from build123d import *
from OCP.BRepFilletAPI import BRepFilletAPI_MakeChamfer

# Parameters (mm, degrees)
EXTRUDE_1_DEPTH  = 8.6
CHAMFER_1_SIZE   = 0.5
CHAMFER_1_SIZE2  = 0.866025404
CHAMFER_2_SIZE   = 0.142054737
CHAMFER_2_SIZE_2 = 0.2


with BuildPart() as part:
    # 草图1 → 凸台-拉伸1 (new body)
    with BuildSketch(Plane.XY):
        with BuildLine():
            Line((-128.840361964, -116.659683115), (-127.425332489, -116.659683115))
            ThreePointArc((-127.425332489, -116.659683115), (-132.090361964, -126.69001389), (-136.755391439, -116.659683115))
            Line((-136.755391439, -116.659683115), (-135.340361964, -116.659683115))
            ThreePointArc((-135.340361964, -116.659683115), (-132.090361964, -125.69001389), (-128.840361964, -116.659683115))
        make_face()
    extrude(amount=EXTRUDE_1_DEPTH)

    # 倒角1: one chamfer whose edges measure the first distance from different faces: ONE call of the kernel's chamfer builder (chamfer() names one face for all edges)
    chamfer_1_edges_1 = [part.edges().sort_by_distance(p)[0] for p in [
        (-136.047876701, -116.659683115, 8.6),
    ]]
    chamfer_1_side_1 = [part.faces().sort_by_distance(p)[0] for p in [
        (-136.047876701, -116.659683115, 4.3),
    ]]
    chamfer_1_edges_2 = [part.edges().sort_by_distance(p)[0] for p in [
        (-128.132847227, -116.659683115, 8.6),
    ]]
    chamfer_1_side_2 = [part.faces().sort_by_distance(p)[0] for p in [
        (-128.132847227, -116.659683115, 4.3),
    ]]
    chamfer_1 = BRepFilletAPI_MakeChamfer(part.part.solid().wrapped)
    for e in chamfer_1_edges_1:
        chamfer_1.Add(CHAMFER_1_SIZE, CHAMFER_1_SIZE2, e.wrapped, chamfer_1_side_1[0].wrapped)  # the first distance lies on this face
    for e in chamfer_1_edges_2:
        chamfer_1.Add(CHAMFER_1_SIZE, CHAMFER_1_SIZE2, e.wrapped, chamfer_1_side_2[0].wrapped)  # the first distance lies on this face
    add(Compound.cast(chamfer_1.Shape()), mode=Mode.REPLACE)

    # 倒角2
    # the kernel refuses this chamfer: 0.2, 0.142054737 mm, written as the material it takes off along each edge
    with BuildSketch(Plane(origin=(-135.340361964, -116.659683115, -0.524920029), x_dir=(-0.7577457918240572, -0.6525498563120925, 0), z_dir=(0, 0, 1))) as chamfer_2_piece_1:
        with BuildLine():
            Line((0.204125918, 0), (CHAMFER_2_SIZE * 0.757745791973, -CHAMFER_2_SIZE * 0.65254985644))
            Line((CHAMFER_2_SIZE * 0.757745791973, -CHAMFER_2_SIZE * 0.65254985644), (0, 0))
            ThreePointArc((0, 0), (0.104949569, -0.001020545), (0.204125918, 0))
        make_face()
    extrude(amount=9.149840059, mode=Mode.SUBTRACT)
    with BuildSketch(Plane(origin=(-128.840361964, -116.659683115, -0.514336598), x_dir=(1, 0, 0), z_dir=(0, 0, 1))) as chamfer_2_piece_2:
        with BuildLine():
            Line((CHAMFER_2_SIZE_2, 0), (0.108073152, -0.091926848))
            ThreePointArc((0.108073152, -0.091926848), (0.054110864, -0.045378858), (0, 0))
            Line((0, 0), (CHAMFER_2_SIZE_2, 0))
        make_face()
    extrude(amount=9.128673195, mode=Mode.SUBTRACT)


solid = part.part
CAD build for the part. Positions are in the model's coordinates, mm. Round coordinates to 2 decimals unless told otherwise and drop trailing zeros. Write each loop counter-clockwise with the first axis right and the second up, starting at its lowest first coordinate (ties: lowest second). Pieces come first, ordered by that corner, then holes. Notation, with made-up numbers: M 19,4.5 L 68,4.5 A27 cw 68,37.5 Z; hole C 46.5,79 d2. An arc over 180 degrees is marked long. Put each result on its own line as item: value. Start each with the question number.
1) Pin check, flat tips, straight feed: pin 1 Ø3 at (x, z) = (-130, 4) entering from -Y; pin 2 Ø1 at (x, z) = (-130.5, 4.5) entering from -Y; pin 3 Ø1 at (y, z) = (-122.5, 6) entering from +X. Stop position of each tip, or through.
2) Pull direction Y, two halves, no side cores. Call faces 1 (the cylindrical face through (-131.896, -126.687, 4.24)), 2 (the flat face through (-127.788, -117.099, 8.354)), 3 (the cylindrical face through (-132.23, -125.69, 4.24)), 4 (the flat face through (-132, -126, 0)): pulls with the +Y half, pulls with the -Y half, needs draft (parallel to the pull), parting line crosses it, or undercut.
3) Saw through at A-A, the plane y = -121.75. Write the cut outline in (x, z), and give its area (3 significant figures).
4) Saw through at D-D, the plane y = -123.75. Write the cut outline in (x, z).
5) Drill centre lines: probe 1 along X at (y, z) = (-120.75, 3); probe 2 along X at (y, z) = (-117.25, 8); probe 3 along Y at (x, z) = (-136.5, 4.25). Where is each one in solid material? Low to high. Write a range as [from, to].
6) Saw through at C-C, the plane x = -136.5. Write the cut outline in (y, z), and give its area (3 significant figures).
7) Saw through at B-B, the plane z = 4.5. Write the cut outline in (x, y), and give its area (3 significant figures).
Resolved:
1. pin 1: y = -126.66
1. pin 2: y = -126.59
1. pin 3: x = -126.16
2. face 1: parting line crosses it
2. face 2: pulls with the +Y half
2. face 3: undercut
2. face 4: needs draft
3. outline: M -138.08,0 L -137.06,0 L -137.06,8.6 L -138.08,8.6 Z; M -127.12,0 L -126.1,0 L -126.1,8.6 L -127.12,8.6 Z
3. area: 17.6 mm²
4. outline: M -137.31,0 L -136.09,0 L -136.09,8.6 L -137.31,8.6 Z; M -128.09,0 L -126.87,0 L -126.87,8.6 L -128.09,8.6 Z
5. probe 1: [-138.19, -137.19], [-126.99, -125.99]
5. probe 2: [-137.19, -135.94], [-128.24, -126.99]
5. probe 3: [-124.8, -123.15], [-118.03, -116.66]
6. outline: M -124.8,0 L -123.15,0 L -123.15,8.6 L -124.8,8.6 Z; M -118.03,0 L -116.66,0 L -116.66,8.1 L -117.53,8.6 L -118.03,8.6 Z
6. area: 25.8 mm²
7. outline: M -136.76,-116.66 A6.1 ccw long -127.43,-116.66 L -128.64,-116.66 L -128.73,-116.75 A5.1 cw long -135.5,-116.79 L -135.48,-116.66 Z
7. area: 26.3 mm²
